```python
from build123d import *

# Parameters (mm, degrees)
BOSS_EXTRUDE1_DEPTH = 25.4
SKETCH2_R           = 2.286
CUT_EXTRUDE1_DEPTH  = 12.43
CUT_EXTRUDE2_DEPTH  = 6.35


with BuildPart() as part:
    # Sketch1 → Boss-Extrude1 (new body)
    with BuildSketch(Plane(origin=(0, 0, 0), x_dir=(0, 0, -1), z_dir=(1, 0, 0))):
        with BuildLine():
            Line((0, 0), (215.9, 0))
            Line((215.9, 0), (185.220791685, 8.220469092))
            ThreePointArc((185.220791685, 8.220469092), (181.900696214, 7.98102699), (179.441604229, 5.73754018))
            ThreePointArc((179.441604229, 5.73754018), (171.472327537, 1.649943093), (164.7682143, 7.58902439))
            ThreePointArc((164.7682143, 7.58902439), (162.965103566, 10.356285306), (159.841631451, 11.43))
            Line((159.841631451, 11.43), (0, 11.43))
            Line((0, 11.43), (0, 0))
        make_face()
    extrude(amount=BOSS_EXTRUDE1_DEPTH)

    # Sketch2 → Cut-Extrude1 (cut, through all)
    with BuildSketch(Plane.XZ):
        with Locations((12.7, -139.7)):
            Circle(SKETCH2_R)
        with Locations((12.7, -88.9)):
            Circle(SKETCH2_R)
        with Locations((12.7, -38.1)):
            Circle(SKETCH2_R)
    extrude(amount=-CUT_EXTRUDE1_DEPTH, mode=Mode.SUBTRACT)

    # Sketch3 → Cut-Extrude2 (cut)
    with BuildSketch(Plane.XZ):
        Polygon((18.12593783, -139.7), (15.412968915, -135.001), (9.987031085, -135.001), (7.27406217, -139.7), (9.987031085, -144.399), (15.412968915, -144.399), align=None)
        Polygon((18.12593783, -88.9), (15.412968915, -84.201), (9.987031085, -84.201), (7.27406217, -88.9), (9.987031085, -93.599), (15.412968915, -93.599), align=None)
        Polygon((18.12593783, -38.1), (15.412968915, -33.401), (9.987031085, -33.401), (7.27406217, -38.1), (9.987031085, -42.799), (15.412968915, -42.799), align=None)
    extrude(amount=-CUT_EXTRUDE2_DEPTH, mode=Mode.SUBTRACT)


solid = part.part
```
Here's how the part is built. I have some questions about the finished solid (model axes, mm). A direction names the side the tool comes from. Round coordinates to 2 decimals unless told otherwise and drop trailing zeros. Write each loop counter-clockwise with the first axis right and the second up, starting at its lowest first coordinate (ties: lowest second). Pieces come first, ordered by that corner, then holes.
Q1. Which directions (+Z, -Z, +X, -X, +Y, -Y) give clear straight access to the entire face, cutting with the end or side of a thin tool? Please do faces 4 (the flat face through (16.8, 3.1, -86.6)), 5 (the cylindrical face through (12.522, 1.634, -171.605)).
Q2. If we section it at C-C on z = -181.5: Write out the boundary of the cut face in (x, y).
Q3. If we mould it in two halves opening along Z, with no side actions, what happens to faces 1 (the flat face through (13, 0, -106)), 2 (the flat face through (12.52, 4.05, -200.78)), 3 (the flat face through (16.75, 3.13, -40.48))? For each: +Z half, -Z half, draft (parallel to the pull), parting line (faces both ways), or undercut.
Q4. Please list where these lines run through material, in increasing order: probe 1 along Z at (x, y) = (12.7, 9.15); probe 2 along Z at (x, y) = (12.7, 10.1); probe 3 along X at (y, z) = (8.4, -139.7).
Q5. Will these pins go through, and if not, where does the flat tip stop? P1, Ø3, axis at x = 4.5, z = -175.5, coming from the +Y side; P2, Ø4.5, axis at x = 12, z = -89, coming from the -Y side.
Q6. If we section it at A-A on y = 3.5: Write out the boundary of the cut face in (x, z).
Answer below:
1. face 4: -Y
1. face 5: +X, -X, +Y
2. outline: (0, 0) - (25.4, 0) - (25.4, 7.79) - (0, 7.79) - close
3. face 1: draft
3. face 2: -Z half
3. face 3: undercut
4. probe 1: z = -164.08 to -141.99, -137.41 to -91.19, -86.61 to -40.39, -35.81 to 0
4. probe 2: z = -163.27 to -141.99, -137.41 to -91.19, -86.61 to -40.39, -35.81 to 0
4. probe 3: x = 0 to 10.41, 14.99 to 25.4
5. P1: stops at y = 3.01
5. P2: stops at y = 6.35
6. outline: (0, -202.84) - (25.4, -202.84) - (25.4, -177.63) - (0, -177.63) - close; (0, -167.3) - (25.4, -167.3) - (25.4, 0) - (0, 0) - close; hole (7.27, -139.7) - (9.99, -144.4) - (15.41, -144.4) - (18.13, -139.7) - (15.41, -135) - (9.99, -135) - close; hole (7.27, -88.9) - (9.99, -93.6) - (15.41, -93.6) - (18.13, -88.9) - (15.41, -84.2) - (9.99, -84.2) - close; hole (7.27, -38.1) - (9.99, -42.8) - (15.41, -42.8) - (18.13, -38.1) - (15.41, -33.4) - (9.99, -33.4) - close
